Check sheet for the drawn part. Datum: minimum x, y, z corner. Units: mm. Give positions to 0.01 mm unless a question says otherwise; leave off trailing zeros. Order: outer loops, then holes, each group sorted by start corner. A loop starts at its lowest first (then second) coordinate and runs counter-clockwise, first axis right, second up. Notation, with made-up numbers: (16.25, 37.5) - (40.25, 37.5) arc R12 ccw to (40.25, 46.5) - close; hole circle Ø5 at (-10, -6.75). An arc over 180 degrees is marked (long way). Answer as a JSON object with one key per item and string values. Group by question number.
(1) Mould release check, pull along X, two halves, no side actions. Record for the marked faces 1, 2, 3 and 4: +X half, -X half, draft (parallel to the pull), parting line (faces both ways), or undercut.
(2) Thickness scan on line 1 (Y direction, x = 4.25, z = 9.5); line 2 (X direction, y = 4.75, z = 13); line 3 (X direction, y = 2.75, z = 0.5). Record the ranges inside material, lowest first.
(3) Section check B-B (x = 3.75). Record the boundary of the cut face in (y, z).
(4) Section check A-A (y = 3). Record the boundary of the cut face in (x, z).
(5) Section check D-D (y = 1.5). Record the boundary of the cut face in (x, z).
(6) Section check C-C (z = 6.75). Record the boundary of the cut face in (x, y), then the cut area to 4 significant figures.
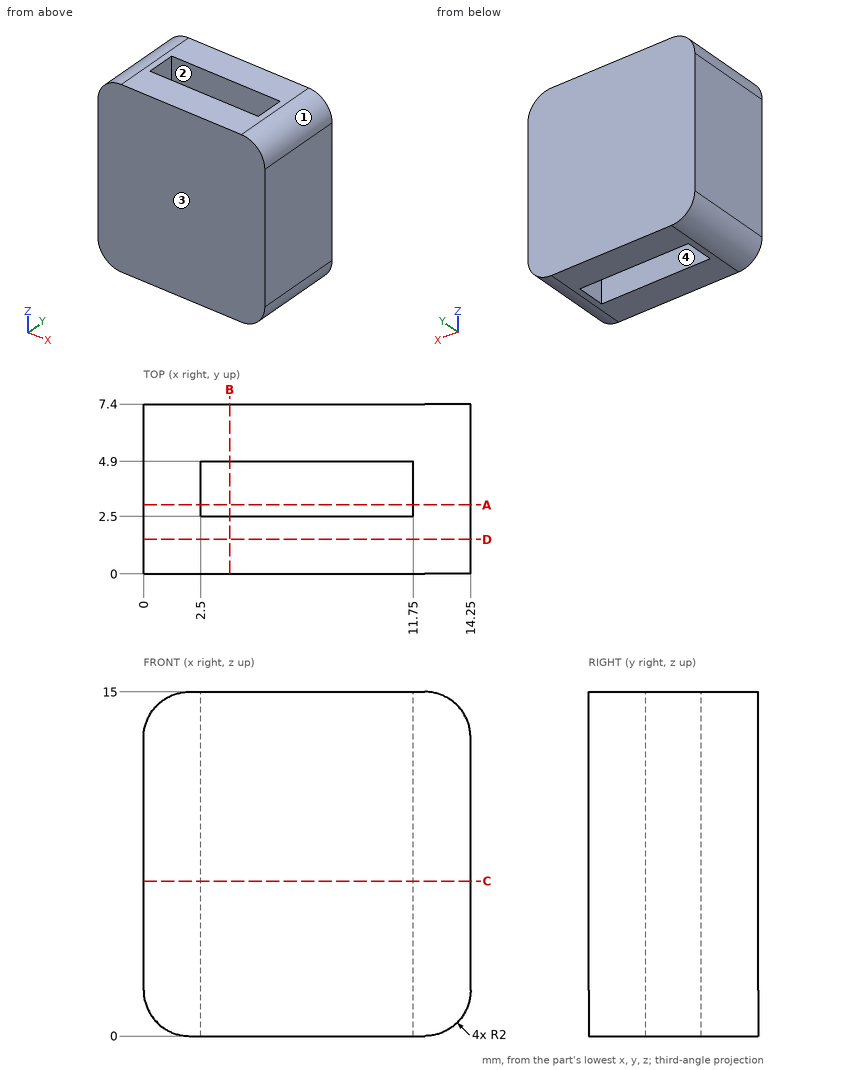
Solutions:
{
 "1": {"face 1": "+X half", "face 2": "undercut", "face 3": "draft", "face 4": "undercut"},
 "2": {"line 1": "y = 0 to 2.5, 4.9 to 7.4", "line 2": "x = 0 to 2.5, 11.75 to 14.25", "line 3": "x = 0.68 to 2.5, 11.75 to 13.57"},
 "3": {"outline": "(0, 0) - (2.5, 0) - (2.5, 15) - (0, 15) - close; (4.9, 0) - (7.4, 0) - (7.4, 15) - (4.9, 15) - close"},
 "4": {"outline": "(0, 2) arc R2 ccw to (2, 0) - (2.5, 0) - (2.5, 15) - (2, 15) arc R2 ccw to (0, 13) - close; (11.75, 0) - (12.25, 0) arc R2 ccw to (14.25, 2) - (14.25, 13) arc R2 ccw to (12.25, 15) - (11.75, 15) - close"},
 "5": {"outline": "(0, 2) arc R2 ccw to (2, 0) - (12.25, 0) arc R2 ccw to (14.25, 2) - (14.25, 13) arc R2 ccw to (12.25, 15) - (2, 15) arc R2 ccw to (0, 13) - close"},
 "6": {"outline": "(0, 0) - (14.25, 0) - (14.25, 7.4) - (0, 7.4) - close; hole (2.5, 2.5) - (11.75, 2.5) - (11.75, 4.9) - (2.5, 4.9) - close", "area": "83.25 mm2"}
}
